```python
from build123d import *

# Parameters (mm, degrees)
SKETCH1_W           = 15
SKETCH1_H           = 15
BOSS_EXTRUDE1_DEPTH = 2
SKETCH4_W           = 1.6
SKETCH4_H           = 3
BOSS_EXTRUDE2_DEPTH = 2


with BuildPart() as part:
    # Sketch1 → Boss-Extrude1 (new body)
    with BuildSketch(Plane(origin=(0, 0, 0), x_dir=(1, 0, 0), z_dir=(0, 1, 0))):
        with Locations((-0.107629188, -0.080708285)):
            Rectangle(SKETCH1_W, SKETCH1_H)
    extrude(amount=BOSS_EXTRUDE1_DEPTH)

    # Sketch4 → Boss-Extrude2 (add)
    with BuildSketch(Plane(origin=(0, 0, 0), x_dir=(1, 0, 0), z_dir=(0, 1, 0))):
        with Locations((3.392370812, -0.080708285)):
            Rectangle(SKETCH4_W, SKETCH4_H)
        with Locations((-3.607629188, -0.080708285)):
            Rectangle(SKETCH4_W, SKETCH4_H)
    extrude(amount=-BOSS_EXTRUDE2_DEPTH)


solid = part.part
```
The listing builds one solid part. Answer for the finished solid, in the listing's coordinates (mm). A direction names the side the tool comes from. Round coordinates to 2 decimals unless told otherwise and drop trailing zeros. Loops run counter-clockwise (first coordinate to the right, second up) from the corner with the lowest first, then second, coordinate; pieces in that order, holes last.
Q1. Section D-D, the plane x = 0 is taken. Determine the outline of the cut face in (y, z).
Q2. For a pull along X with two mould halves and no side action, classify faces 6 (the face through (-2.808, -1, 0)), 7 (the face through (-4.408, -1, 0)), 8 (the face through (3, -1, -1.419)) as released by +X, released by -X, zero draft, split by the parting line, or undercut.
Q3. Section A-A, the plane y = -0.3 is taken. Determine the outline of the cut face in (x, z).
Q4. Section C-C, the plane z = 1.25 is taken. Determine the outline of the cut face in (x, y), then the cut area to 3 significant figures.
Q5. Given pin 1 Ø1.3 at (x, y) = (3.5, -1) entering from +Z; pin 2 Ø1 at (y, z) = (-1.5, -0.5) entering from +X; pin 3 Ø1.3 at (x, y) = (-3.5, -1) entering from -Z, each flat-ended and moving along its own axis, determine where each tip first touches the part or whether it passes through.
Q6. Section B-B, the plane x = 4 is taken. Determine the outline of the cut face in (y, z), then the cut area to 3 significant figures.
Q7. Find the intervals of material crossed by line 1 (X direction, y = -0.6, z = -0.75); line 2 (Y direction, x = 3.75, z = 3.5); line 3 (Z direction, x = 3, y = -1), in increasing order.
Q8. Which of the six approach directions +Z, -Z, +X, -X, +Y, -Y give full straight-line access (tool end or side, diameter ignored) to faces 1 (the face through (-4, -1, -1.419)), 2 (the face through (4.192, -1, 0)), 3 (the face through (2.592, -1, 0)), 4 (the face through (3, -1, 1.581)), 5 (the face through (0, 1, 7.581))?
Completed:
1. outline: (0, -7.42) - (2, -7.42) - (2, 7.58) - (0, 7.58) - close
2. face 6: undercut
2. face 7: released by -X
2. face 8: zero draft
3. outline: (-4.41, -1.42) - (-2.81, -1.42) - (-2.81, 1.58) - (-4.41, 1.58) - close; (2.59, -1.42) - (4.19, -1.42) - (4.19, 1.58) - (2.59, 1.58) - close
4. outline: (-7.61, 0) - (-4.41, 0) - (-4.41, -2) - (-2.81, -2) - (-2.81, 0) - (2.59, 0) - (2.59, -2) - (4.19, -2) - (4.19, 0) - (7.39, 0) - (7.39, 2) - (-7.61, 2) - close
4. area: 36.4 mm2
5. pin 1: stops at z = 1.58
5. pin 2: stops at x = 4.19
5. pin 3: stops at z = -1.42
6. outline: (-2, -1.42) - (0, -1.42) - (0, -7.42) - (2, -7.42) - (2, 7.58) - (0, 7.58) - (0, 1.58) - (-2, 1.58) - close
6. area: 36.0 mm2
7. line 1: x = -4.41 to -2.81, 2.59 to 4.19
7. line 2: y = 0 to 2
7. line 3: z = -1.42 to 1.58
8. face 1: -Z, +X, -X, -Y
8. face 2: +Z, -Z, +X, -Y
8. face 3: +Z, -Z, -Y
8. face 4: +Z, +X, -X, -Y
8. face 5: +Z, +X, -X, +Y, -Y
